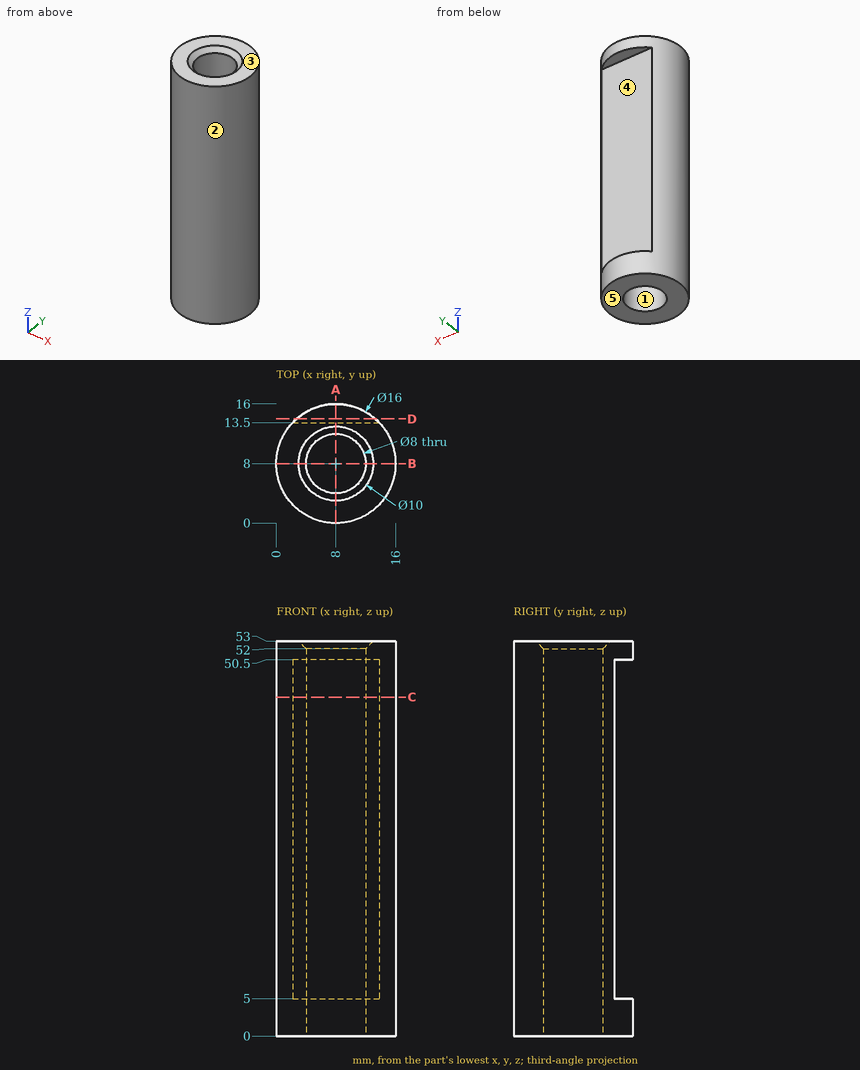
For this review, use the dimensioned drawing (mm, ordinates from the lowest corner) and the shaded views. A direction names the side the tool comes from. Give positions to 0.01 mm unless a question says otherwise; leave off trailing zeros. Order: outer loops, then holes, each group sorted by start corner. A loop starts at its lowest first (then second) coordinate and runs counter-clockwise, first axis right, second up. Notation, with made-up numbers: M 45.5,-6 L 62.5,-6 A23 ccw 62.5,15 Z; hole C 68.5,19.25 d1. An arc over 180 degrees is marked long. Use one line per item in the form item = value. Start each with the question number.
Item 1: Insertion check: pin 1 Ø6.5 at (x, y) = (8, 8) entering from -Z; pin 2 Ø3.5 at (x, z) = (8.5, 37.5) entering from +Y; pin 3 Ø1.5 at (y, z) = (6, 12) entering from +X. Each pin has a flat end and moves straight along its axis. Give the tip position at first contact, or say it passes through.
Item 2: We need section C-C on z = 45.5. Give the boundary of the cut face in (x, y), plus the area to 3 significant figures.
Item 3: We need section D-D on y = 14. Give the boundary of the cut face in (x, z).
Item 4: We need section A-A on x = 8. Give the boundary of the cut face in (y, z).
Item 5: The part is to be moulded in two halves that separate along X. For the marked faces 1, 2 and 3, say which applies: pulls with the +X half, pulls with the -X half, needs draft (parallel to the pull), parting line crosses it, or undercut.
Item 6: For the marked faces 4 and 5, list the 3-axis set-ups (+Z, -Z, +X, -X, +Y, -Y) from which the entire face can be reached by the end or side of a thin tool; tool diameter is ignored.
Item 7: To check wall thickness, follow line 1 along X through (y, z) = (8, 22.5); line 2 along Z through (x, y) = (6.25, 14.5); line 3 along Y through (x, z) = (8, 15). State the ranges of each line that lie inside material, in increasing order. Write a range as from..to.
Item 8: We need section B-B on y = 8. Give the boundary of the cut face in (x, z), plus the area to 3 significant figures.
Completed:
q1.pin_1 = through
q1.pin_2 = 13.5
q1.pin_3 = 15.9
q2.outline = M 2.19,13.5 A8 ccw long 13.81,13.5 Z; hole C 8,8 d8
q2.area = 131 mm²
q3.outline = M 2.71,0 L 13.29,0 L 13.29,5 L 2.71,5 Z; M 2.71,50.5 L 13.29,50.5 L 13.29,53 L 2.71,53 Z
q4.outline = M 0,0 L 4,0 L 4,52 L 3,53 L 0,53 Z; M 12,0 L 16,0 L 16,5 L 13.5,5 L 13.5,50.5 L 16,50.5 L 16,53 L 13,53 L 12,52 Z
q5.face_1 = undercut
q5.face_2 = parting line crosses it
q5.face_3 = needs draft
q6.face_4 = +X, -X, +Y
q6.face_5 = -Z, +X, -X, +Y, -Y
q7.line_1 = 0..4, 12..16
q7.line_2 = 0..5, 50.5..53
q7.line_3 = 0..4, 12..13.5
q8.outline = M 0,0 L 4,0 L 4,52 L 3,53 L 0,53 Z; M 12,0 L 16,0 L 16,53 L 13,53 L 12,52 Z
q8.area = 423 mm²
